CAD build for the part. Positions are in the model's coordinates, mm. Coordinates: 2 decimals unless noted, no trailing zeros. Loops run counter-clockwise (first coordinate to the right, second up) from the corner with the lowest first, then second, coordinate; pieces in that order, holes last. Notation, with made-up numbers: (-14.75, 9.25) - (28.25, 9.25) arc R37 cw to (28.25, 45.25) - close; hole circle Ø9 at (-33, -27). An arc over 180 degrees is marked (long way). Put each result on its own line as item: value.
```python
from build123d import *

# Parameters (mm, degrees)
SKETCH_1_R      = 2.75
EXTRUDE_1_DEPTH = 89
SKETCH_2_R      = 2
EXTRUDE_2_DEPTH = 13
SKETCH_3_R      = 1.5
EXTRUDE_3_DEPTH = 5


with BuildPart() as part:
    # 草图1 → 凸台-拉伸1 (new body)
    with BuildSketch(Plane.XY):
        Circle(SKETCH_1_R)
    extrude(amount=EXTRUDE_1_DEPTH)

    # 草图2 → 凸台-拉伸2 (add)
    with BuildSketch(Plane.XY.offset(89)):
        with Locations(Location((0, 0, 0), (0, 0, 180))):
            Circle(SKETCH_2_R)
    extrude(amount=EXTRUDE_2_DEPTH)

    # 草图3 → 凸台-拉伸3 (add)
    with BuildSketch(Plane.XY.offset(102)):
        Circle(SKETCH_3_R)
    extrude(amount=EXTRUDE_3_DEPTH)

    # 草图4 → 旋转1 (revolve)
    with BuildSketch(Plane(origin=(0, 0, 0), x_dir=(1, 0, 0), z_dir=(0, 1, 0))):
        Polygon((0, -107), (0, -108.500036411), (-1.5, -107), align=None)
    revolve(axis=Axis((0, 0, 107), (0, 0, 1)))


solid = part.part
```
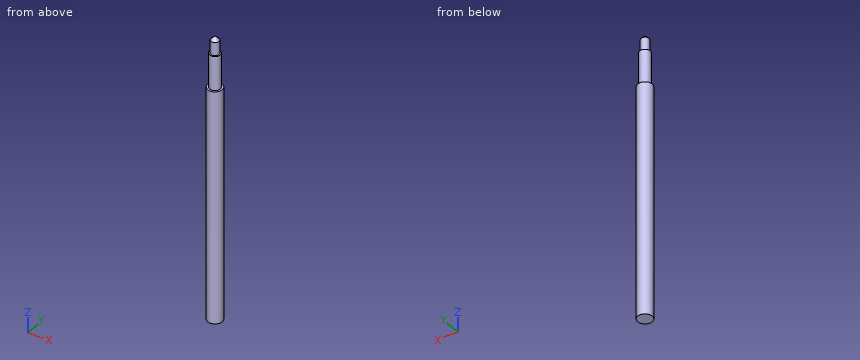
Q1. Wall check: L1, parallel to X at y = 2.3, z = 47; L2, parallel to Z at x = -2.25, y = -0.9; L3, parallel to X at y = -0.15, z = 97. Give the ranges that are in metal, low to high. Write a range as from..to.
Determined:
L1: -1.51..1.51
L2: 0..89
L3: -1.99..1.99
Q2. Slice it at B-B, the plane z = 31.5. Give the cut face in (x, y), then the cut area to 3 significant figures.
Determined:
outline: circle Ø5.5 at (0, 0)
area: 23.8 mm2
Q3. Pin check, flat tips, straight feed: pin 1 Ø1 at (x, z) = (2, 52.5) entering from +Y; pin 2 Ø1.5 at (x, z) = (-1, 58) entering from +Y. Stop position of each tip, or through.
Determined:
pin 1: y = 2.3
pin 2: y = 2.74
Q4. Slice it at A-A, the plane z = 92.5. Give the cut face in (x, y).
Determined:
outline: circle Ø4 at (0, 0)
